from build123d import *

# Parameters (mm, degrees)
F1_DEPTH = 1.778
F2_DEPTH = 1.5748
F3_DEPTH = 1.778


with BuildPart() as f1:
    # F0 (on Front) → F1 (new body)
    with BuildSketch(Plane.XZ):
        with BuildLine():
            Line((14.02935353, 41.1213250894), (16.2583384663, 59.9522180855))
            ThreePointArc((16.2583384663, 59.9522180855), (-0.9637356423, 76.1819680311), (-16.1440849231, 58.0281360497))
            Line((-16.1440849231, 58.0281360497), (-14.1149313353, 41.0024441959))
            Line((-14.1149313353, 41.0024441959), (-1.6278814086, -63.7706323678))
            Line((-1.6278814086, -63.7706323678), (-1.5574045531, -64.3619711562))
            Line((-1.5574045531, -64.3619711562), (-0.1437664474, -76.223156493))
            ThreePointArc((-0.1437664474, -76.223156493), (-0.0022464, -76.237388177), (0.1393582085, -76.2240240658))
            Line((0.1393582085, -76.2240240658), (1.5482228022, -64.3216652936))
            Line((1.5482228022, -64.3216652936), (14.02935353, 41.1213250894))
        make_face()
    extrude(amount=F1_DEPTH)

    # F2 (add): a face of the model
    f2_faces = [f1.faces().sort_by_distance(p)[0] for p in [
        (-0.03237785, 0, 22.4036287073),
    ]]
    extrude(f2_faces, amount=F2_DEPTH)

    # F0 (on Front) → F3 (join)
    with BuildSketch(Plane.XZ):
        with BuildLine():
            ThreePointArc((19.465577211, 35.0036723741), (17.9101589408, 39.0956829635), (14.02935353, 41.1213250894))
            Line((14.02935353, 41.1213250894), (1.5482228022, -64.3216652936))
            ThreePointArc((1.5482228022, -64.3216652936), (1.9456415345, -64.2155103566), (2.1613873882, -63.865275798))
            ThreePointArc((2.1613873882, -63.865275798), (2.1676286256, -63.8175184176), (2.1697142526, -63.7694001198))
            Line((2.1697142526, -63.7694001198), (2.1781676915, -63.7694001198))
            Line((2.1781676915, -63.7694001198), (19.465577211, 35.0036723741))
        make_face()
        with BuildLine():
            Line((-1.6278814086, -63.7706323678), (-14.1149313353, 41.0024441959))
            ThreePointArc((-14.1149313353, 41.0024441959), (-18.2559821933, 38.6033472019), (-19.3598979472, 33.9465952648))
            Line((-19.3598979472, 33.9465952648), (-2.2124765092, -63.7709956311))
            ThreePointArc((-2.2124765092, -63.7709956311), (-2.0162187298, -64.2119998537), (-1.5574045531, -64.3619711562))
            Line((-1.5574045531, -64.3619711562), (-1.6278814086, -63.7706323678))
        make_face()
    extrude(amount=F3_DEPTH)


solid = f1.part
Work out the finished part from the listing and answer in its coordinate system (mm). A direction names the side the tool comes from. Give positions to 0.01 mm unless a question says otherwise; leave off trailing zeros. Loops run counter-clockwise (first coordinate to the right, second up) from the corner with the lowest first, then second, coordinate; pieces in that order, holes last. Notation, with made-up numbers: (30.25, 47) - (37.25, 47) arc R11 cw to (37.25, 53) - close; hole circle Ø10 at (20, 56.25). An arc over 180 degrees is marked (long way). Answer in a Markdown table with one row per item. Add a question column.
Q1. Determine the mould class of faces 3 (the cylindrical face through (17.95, -0.88, 39.05)), 4 (the flat face through (-12, 0, 0)), 5 (the flat face through (10.7, -0.88, -15.07)) for opening direction Z: released by +Z, released by -Z, zero draft, split by the parting line, or undercut.
Q2. Each of these flat-tipped pins is pushed along its axis until it touches: P1, Ø3, axis at x = -14, z = 2, coming from the +Y side; P2, Ø1, axis at x = -12, z = -12.5, coming from the +Y side; P3, Ø19.5, axis at x = 8, z = -12.5, coming from the +Y side; P4, Ø1.5, axis at y = 0.5, z = -41, coming from the -X side. Where does it stop, or does it pass through?
Q3. The part is cut by section B-B (z = 8). Determine the outline of the cut face in (x, y), and give its area (3 significant figures).
Q4. The part is cut by section D-D (x = 12). Determine the outline of the cut face in (y, z), and give its area (3 significant figures).
Q5. The part is cut by section C-C (x = 4). Determine the outline of the cut face in (y, z).
Q6. A tool of negligible diameter and unlimited length cuts with its end or side. For faces 1 (the cylindrical face through (-18.215, -0.877, 38.658)), 2 (the flat face through (11, 0, 0)), from which of +Z, -Z, +X, -X, +Y, -Y can it reach the whole face along a straight path? Write none if from no direction.
Q7. The part is cut by section A-A (y = 0.6). Determine the outline of the cut face in (x, z).
Q8. Consider line 1 along Y through (x, z) = (-14, 24.5); line 2 along X through (y, z) = (0.55, 51.5); line 3 along X through (y, z) = (0.6, -38). Determine where each line is inside the solid, lowest interval first.
Solution:
| question | item | result |
|---|---|---|
| 1 | face 3 | undercut |
| 1 | face 4 | zero draft |
| 1 | face 5 | released by -Z |
| 2 | P1 | stops at y = 0 |
| 2 | P2 | passes through |
| 2 | P3 | stops at y = 1.57 |
| 2 | P4 | stops at x = -6.31 |
| 3 | outline | (-14.81, -1.78) - (14.74, -1.78) - (14.74, 0) - (10.11, 0) - (10.11, 1.57) - (-10.18, 1.57) - (-10.18, 0) - (-14.81, 0) - close |
| 3 | area | 84.5 mm² |
| 4 | outline | (-1.78, -7.65) - (0, -7.65) - (0, 23.98) - (1.57, 23.98) - (1.57, 70.92) - (-1.78, 70.92) - close |
| 4 | area | 214 mm² |
| 5 | outline | (-1.78, -53.36) - (0, -53.36) - (0, -43.61) - (1.57, -43.61) - (1.57, 75.71) - (-1.78, 75.71) - close |
| 6 | face 1 | -X, +Y, -Y |
| 6 | face 2 | -Z, +X, +Y |
| 7 | outline | (-16.14, 58.03) - (-0.14, -76.22) arc R0.73 ccw to (0.14, -76.22) - (16.26, 59.95) arc R16.26 ccw (long way) to start |
| 8 | line 1 | y = -1.78 to 0 |
| 8 | line 2 | x = -15.37 to 15.26 |
| 8 | line 3 | x = -4.7 to 4.66 |
